Read the model definition and answer for the solid it produces. Units are mm, in the model's axes. A direction names the side the tool comes from. Give positions to 0.01 mm unless a question says otherwise; leave off trailing zeros. Order: outer loops, then holes, each group sorted by start corner. A loop starts at its lowest first (then second) coordinate and runs counter-clockwise, first axis right, second up. Notation, with made-up numbers: M -36,44.25 L -4,44.25 A33 ccw -4,77.25 Z; hole C -16.75,78.25 d11. An arc over 180 degrees is marked long. One line per item, written item: value. Start each with the question number.
from build123d import *

# Parameters (mm, degrees)
SKETCH1_W           = 5.9944
SKETCH1_H           = 5.9944
BOSS_EXTRUDE1_DEPTH = 8.5852
SKETCH3_R           = 2.54
BOSS_EXTRUDE2_DEPTH = 0.8509
SKETCH4_R           = 1.93675
BOSS_EXTRUDE3_DEPTH = 9.5885
BOSS_EXTRUDE4_DEPTH = 5.9563
SKETCH6_R           = 3.8481
BOSS_EXTRUDE5_DEPTH = 2.54
SKETCH7_R           = 3.2512
CUT_EXTRUDE1_DEPTH  = 2.54


with BuildPart() as part:
    # Sketch1 → Boss-Extrude1 (new body)
    with BuildSketch(Plane(origin=(0, 0, 0), x_dir=(1, 0, 0), z_dir=(0, 1, 0))):
        Rectangle(SKETCH1_W, SKETCH1_H)
    extrude(amount=BOSS_EXTRUDE1_DEPTH)

    # Sketch2 → Cut-Revolve1 (revolve, cut)
    with BuildSketch(Plane.XY):
        Polygon((2.8956, 1.6129), (2.8956, 0), (5.460904916, -1.481079484), (5.460904916, 3.093979484), align=None)
        Polygon((2.9972, 8.5852), (2.8956, 8.5852), (5.460904916, 7.104120516), (5.460904916, 8.5852), align=None)
    revolve(axis=Axis((0, 0.80645, 0), (0, 1, 0)), mode=Mode.SUBTRACT)

    # Sketch3 → Boss-Extrude2 (add)
    with BuildSketch(Plane(origin=(0, 0, -2.9972), x_dir=(-1, 0, 0), z_dir=(0, 0, -1))):
        with Locations(Location((0, 5.09905, 0), (0, 0, 180))):
            Circle(SKETCH3_R)
    extrude(amount=BOSS_EXTRUDE2_DEPTH)

    # Sketch4 → Boss-Extrude3 (add)
    with BuildSketch(Plane(origin=(0, 0, -3.8481), x_dir=(-1, 0, 0), z_dir=(0, 0, -1))):
        with Locations(Location((0, 5.09905, 0), (0, 0, 180))):
            Circle(SKETCH4_R)
    extrude(amount=BOSS_EXTRUDE3_DEPTH)

    # Sketch5 → Boss-Extrude4 (add)
    with BuildSketch(Plane(origin=(0, 0, 0), x_dir=(-1, 0, 0), z_dir=(0, -1, 0))):
        Polygon((0, 4.59005011), (-3.9751, 2.295025055), (-3.9751, -2.295025055), (0, -4.59005011), (3.9751, -2.295025055), (3.9751, 2.295025055), align=None)
    extrude(amount=BOSS_EXTRUDE4_DEPTH)

    # Sketch6 → Boss-Extrude5 (add)
    with BuildSketch(Plane(origin=(0, -5.9563, 0), x_dir=(-1, 0, 0), z_dir=(0, -1, 0))):
        with Locations(Location((0, 0, 0), (0, 0, 90))):
            Circle(SKETCH6_R)
    extrude(amount=BOSS_EXTRUDE5_DEPTH)

    # Sketch7 → Cut-Extrude1 (cut)
    with BuildSketch(Plane(origin=(0, -8.4963, 0), x_dir=(-1, 0, 0), z_dir=(0, -1, 0))):
        with Locations(Location((0, 0, 0), (0, 0, 90))):
            Circle(SKETCH7_R)
    extrude(amount=-CUT_EXTRUDE1_DEPTH, mode=Mode.SUBTRACT)


solid = part.part
Q1. Consider probe 1 along X at (y, z) = (-7.15, 0); probe 2 along Z at (x, y) = (0.5, 2); probe 3 along X at (y, z) = (-6.25, 0.25). Determine where each line is inside the solid, lowest interval first.
Q2. Determine the mould class of faces 1 (the flat face through (3, -8.496, 2)), 2 (the flat face through (-3.975, -3, 0)), 3 (the flat face through (2.997, 5, 0)), 4 (the flat face through (0, -5.956, 0)) for opening direction X: released by +X, released by -X, zero draft, split by the parting line, or undercut.
Q3. Find section B-B, the plane x = 3.5. Give the vertices of the cut face in (y, z).
Q4. A tool of negligible diameter and unlimited length cuts with its end or side. For faces 5 (the flat face through (1, 0, 3)), 6 (the cylindrical face through (3.815, -7.209, 0.501)), 7 (the cylindrical face through (-0.33, 2.58, -3.42)), from which of +Z, -Z, +X, -X, +Y, -Y can it reach the whole face along a straight path? Write none if from no direction.
Q5. Find section C-C, the plane z = -12.25. Give the vertices of the cut face in (x, y), then the cut area to 3 significant figures.
Q6. Each of these flat-tipped pins is pushed along its axis until it touches: pin 1 (4 mm diameter, centred on x = -0.5, z = -6, fed in from +Y); pin 2 (3 mm diameter, centred on y = 6, z = 0.5, fed in from -X); pin 3 (1.5 mm diameter, centred on x = -1.5, z = -10, fed in from -Y). Where does it stop, or does it pass through?
Q7. Find section D-D, the plane y = 6.75. Give the vertices of the cut face in (x, z), then the cut area to 3 significant figures.
Q8. Find section A-A, the plane y = -0.5. Give the vertices of the cut face in (x, z), then the cut area to 3 significant figures.
Evaluation:
1. probe 1: -3.85 to -3.25, 3.25 to 3.85
1. probe 2: -3 to 3
1. probe 3: -3.84 to -3.24, 3.24 to 3.84
2. face 1: zero draft
2. face 2: released by -X
2. face 3: released by +X
2. face 4: undercut
3. outline: M -8.5,-1.6 L -5.96,-1.6 L -5.96,-2.57 L 0,-2.57 L 0,2.57 L -5.96,2.57 L -5.96,1.6 L -8.5,1.6 Z
4. face 5: none
4. face 6: -Y
4. face 7: -Z
5. outline: C 0,5.1 d3.87
5. area: 11.8 mm2
6. pin 1: y = 7.04
6. pin 2: x = -3
6. pin 3: y = 3.31
7. outline: M -3,-3 L -1.93,-3 L -1.93,-3.85 L -1.01,-3.85 L -1.01,-13.44 L 1.01,-13.44 L 1.01,-3.85 L 1.93,-3.85 L 1.93,-3 L 3,-3 L 3,3 L -3,3 Z
7. area: 58.6 mm2
8. outline: M -3.98,-2.3 L 0,-4.59 L 3.98,-2.3 L 3.98,2.3 L 0,4.59 L -3.98,2.3 Z
8. area: 54.7 mm2
